Here's how the part is built. I have some questions about the finished solid (model axes, mm). A direction names the side the tool comes from. Round coordinates to 2 decimals unless told otherwise and drop trailing zeros. Loops run counter-clockwise (first coordinate to the right, second up) from the corner with the lowest first, then second, coordinate; pieces in that order, holes last. Notation, with made-up numbers: M 11.25,-23.75 L 42.25,-23.75 A27 ccw 42.25,-6.75 Z; hole C 71,29 d11. An arc over 180 degrees is marked long. Use a Markdown table: item, result.
```python
from build123d import *

# Parameters (mm, degrees)
SKETCH1_R           = 1.55
BOSS_EXTRUDE1_DEPTH = 1.6
SKETCH2_W           = 25.9
SKETCH2_H           = 2.35
SKETCH2_W_2         = 20.8
SKETCH2_W_3         = 15.75
SKETCH2_W_4         = 4.95
SKETCH2_H_2         = 7.3
BOSS_EXTRUDE2_DEPTH = 8.7
SKETCH3_W           = 16.15
SKETCH3_H           = 12.5
SKETCH3_W_2         = 14.4
SKETCH3_H_2         = 8.9
BOSS_EXTRUDE3_DEPTH = 10.6


with BuildPart() as part:
    # Sketch1 → Boss-Extrude1 (new body)
    with BuildSketch(Plane(origin=(0, 0, 0), x_dir=(1, 0, 0), z_dir=(0, 1, 0))):
        Polygon((66, 52.297918472), (66, 39.5), (68.5, 37), (68.5, 4.5), (66, 2), (66, 0), (0, 0), (0, 53.5), (64.797918472, 53.5), align=None)
        with Locations((15, 51.1)):
            Circle(SKETCH1_R, mode=Mode.SUBTRACT)
        with Locations((66.1, 35.9)):
            Circle(SKETCH1_R, mode=Mode.SUBTRACT)
        with Locations((66.1, 7.7)):
            Circle(SKETCH1_R, mode=Mode.SUBTRACT)
        with Locations((13.85, 2.4)):
            Circle(SKETCH1_R, mode=Mode.SUBTRACT)
    extrude(amount=BOSS_EXTRUDE1_DEPTH)

    # Sketch2 → Boss-Extrude2 (add)
    with BuildSketch(Plane(origin=(0, 1.6, 0), x_dir=(1, 0, 0), z_dir=(0, 1, 0))):
        with Locations((30.15, 51.025)):
            Rectangle(SKETCH2_W, SKETCH2_H)
        with Locations((54.7, 51.025)):
            Rectangle(SKETCH2_W_2, SKETCH2_H)
        with Locations((57.378669226, 2.475)):
            Rectangle(SKETCH2_W_3, SKETCH2_H)
        with Locations((36.953669226, 2.475)):
            Rectangle(SKETCH2_W_2, SKETCH2_H)
        with Locations((64.725, 28.45)):
            Rectangle(SKETCH2_W_4, SKETCH2_H_2)
    extrude(amount=BOSS_EXTRUDE2_DEPTH)

    # Sketch3 → Boss-Extrude3 (add)
    with BuildSketch(Plane(origin=(0, 1.6, 0), x_dir=(1, 0, 0), z_dir=(0, 1, 0))):
        with Locations((1.825, 38.35)):
            Rectangle(SKETCH3_W, SKETCH3_H)
        with Locations((5.8, 8.15)):
            Rectangle(SKETCH3_W_2, SKETCH3_H_2)
    extrude(amount=BOSS_EXTRUDE3_DEPTH)


solid = part.part
```
Q1. I need wall thicknesses on line 1 (Z direction, x = 56, y = 9.5); line 2 (X direction, y = 0.9, z = -7.7); line 3 (X direction, y = 0.6, z = -51.1). Which ranges of each line are inside material? Lowest first, please. Write a range as from..to.
Return value:
| item | result |
|---|---|
| line 1 | z = -52.2..-49.85, -3.65..-1.3 |
| line 2 | x = 0..64.55, 67.65..68.5 |
| line 3 | x = 0..13.45, 16.55..66 |
Q2. Will these pins go through, and if not, where does the flat tip stop? P1, Ø5.5, axis at y = 4.5, z = -41, coming from the +X side; P2, Ø2.5, axis at x = 36, y = 4.5, coming from the -Z side; P3, Ø1.9, axis at y = 7.5, z = -2.5, coming from the +X side.
Return value:
| item | result |
|---|---|
| P1 | stops at x = 9.9 |
| P2 | stops at z = -52.2 |
| P3 | stops at x = 65.25 |
Q3. Imagine slicing it at C-C, the plane x = 1. Please give me the cut outline in (y, z), then the cut area to 3 significant figures.
Return value:
| item | result |
|---|---|
| outline | M 0,-53.5 L 1.6,-53.5 L 1.6,-44.6 L 12.2,-44.6 L 12.2,-32.1 L 1.6,-32.1 L 1.6,-12.6 L 12.2,-12.6 L 12.2,-3.7 L 1.6,-3.7 L 1.6,0 L 0,0 Z |
| area | 312 mm^2 |
Q4. For faces 1 (the flat face through (55, 6, -49.85)), 2 (the flat face through (17.2, 6, -51)), 3 (the flat face through (-1, 1.6, -8)), 4 (the flat face through (2, 7, -32.1)), which set-ups out of +Z, -Z, +X, -X, +Y, -Y let a thin tool reach every point of the face, with its end or its side?
Return value:
| item | result |
|---|---|
| face 1 | +X, -X, +Y |
| face 2 | +Z, -Z, -X, +Y |
| face 3 | +Z, -Z, -X, -Y |
| face 4 | -X, +Y |
Q5. Imagine slicing it at D-D, the plane z = -42.5. Please give me the cut outline in (x, y), then the cut area to 3 significant figures.
Return value:
| item | result |
|---|---|
| outline | M -6.25,1.6 L 0,1.6 L 0,0 L 66,0 L 66,1.6 L 9.9,1.6 L 9.9,12.2 L -6.25,12.2 Z |
| area | 277 mm^2 |
Q6. Imagine slicing it at B-B, the plane z = -7.7. Please give me the cut outline in (x, y), then the cut area to 3 significant figures.
Return value:
| item | result |
|---|---|
| outline | M -1.4,1.6 L 0,1.6 L 0,0 L 64.55,0 L 64.55,1.6 L 13,1.6 L 13,12.2 L -1.4,12.2 Z; M 67.65,0 L 68.5,0 L 68.5,1.6 L 67.65,1.6 Z |
| area | 257 mm^2 |
Q7. Imagine slicing it at A-A, the plane y = 9.25. Please give me the cut outline in (x, z).
Return value:
| item | result |
|---|---|
| outline | M -6.25,-44.6 L 9.9,-44.6 L 9.9,-32.1 L -6.25,-32.1 Z; M -1.4,-12.6 L 13,-12.6 L 13,-3.7 L -1.4,-3.7 Z; M 17.2,-52.2 L 43.1,-52.2 L 43.1,-49.85 L 17.2,-49.85 Z; M 26.55,-3.65 L 47.35,-3.65 L 47.35,-1.3 L 26.55,-1.3 Z; M 44.3,-52.2 L 65.1,-52.2 L 65.1,-49.85 L 44.3,-49.85 Z; M 49.5,-3.65 L 65.25,-3.65 L 65.25,-1.3 L 49.5,-1.3 Z; M 62.25,-32.1 L 67.2,-32.1 L 67.2,-24.8 L 62.25,-24.8 Z |
Q8. We'd pull the mould along X, two halves only. Please class faces 5 (the flat face through (-3, 1.6, -38)), 6 (the flat face through (62.25, 6, -28)), 7 (the cylindrical face through (67.578, 0.789, -8.166)), 8 (the flat face through (66, 1, -1)): pulls with the +X half, pulls with the -X half, needs draft (parallel to the pull), parting line crosses it, or undercut.
Return value:
| item | result |
|---|---|
| face 5 | needs draft |
| face 6 | pulls with the -X half |
| face 7 | undercut |
| face 8 | pulls with the +X half |
